from build123d import *

# Parameters (mm, degrees)
F0_R     = 2.5
F1_DEPTH = 15
F0_R_2   = 5
F0_R_3   = 3.5
F2_DEPTH = 2.5
F3_DEPTH = 9.5
F4_R     = 0.5
F5_R     = 0.5


with BuildPart() as f1:
    # F0 (on Front) → F1 (new body)
    with BuildSketch(Plane.XZ):
        Circle(F0_R)
    extrude(amount=F1_DEPTH)

    # F0 (on Front) → F2 (join)
    with BuildSketch(Plane.XZ):
        Circle(F0_R_2)
        Circle(F0_R_3, mode=Mode.SUBTRACT)
        Circle(F0_R_3)
        Circle(F0_R, mode=Mode.SUBTRACT)
        Circle(F0_R)
    extrude(amount=-F2_DEPTH)

    # F0 (on Front) → F3 (join)
    with BuildSketch(Plane.XZ):
        Circle(F0_R_3)
        Circle(F0_R, mode=Mode.SUBTRACT)
        Circle(F0_R)
    extrude(amount=-F3_DEPTH)

    # F4
    f4_edges = [f1.edges().sort_by_distance(p)[0] for p in [
        (-3.5, 9.5, 0),
    ]]
    fillet(f4_edges, radius=F4_R)

    # F5
    f5_edges = [f1.edges().sort_by_distance(p)[0] for p in [
        (-2.5, -15, 0),
    ]]
    fillet(f5_edges, radius=F5_R)


solid = f1.part
Check sheet for the modelled part. Datum: model origin and axes. Units: mm. A direction names the side the tool comes from. Coordinates: 2 decimals unless noted, no trailing zeros. Loops run counter-clockwise (first coordinate to the right, second up) from the corner with the lowest first, then second, coordinate; pieces in that order, holes last. Notation, with made-up numbers: (66, 30.25) -> (112, 30.25) arc R21 ccw to (112, 42.25) -> close; hole circle Ø6 at (-27, -1). An arc over 180 degrees is marked (long way). Answer in a Markdown table with one row per item.
1. Sectioned sample at A-A, the plane z = 0. Record the boundary of the cut face in (x, y).
Check values:
| item | result |
|---|---|
| outline | (-5, 0) -> (-2.5, 0) -> (-2.5, -14.5) arc R0.5 ccw to (-2, -15) -> (2, -15) arc R0.5 ccw to (2.5, -14.5) -> (2.5, 0) -> (5, 0) -> (5, 2.5) -> (3.5, 2.5) -> (3.5, 9) arc R0.5 ccw to (3, 9.5) -> (-3, 9.5) arc R0.5 ccw to (-3.5, 9) -> (-3.5, 2.5) -> (-5, 2.5) -> close |
2. Sectioned sample at B-B, the plane x = 0. Record the boundary of the cut face in (y, z).
Check values:
| item | result |
|---|---|
| outline | (-15, -2) arc R0.5 ccw to (-14.5, -2.5) -> (0, -2.5) -> (0, -5) -> (2.5, -5) -> (2.5, -3.5) -> (9, -3.5) arc R0.5 ccw to (9.5, -3) -> (9.5, 3) arc R0.5 ccw to (9, 3.5) -> (2.5, 3.5) -> (2.5, 5) -> (0, 5) -> (0, 2.5) -> (-14.5, 2.5) arc R0.5 ccw to (-15, 2) -> close |
3. Go/stop test with flat-tipped pins: pin 1 (1 mm diameter, centred on y = -4.5, z = 2, fed in from +X); pin 2 (2 mm diameter, centred on y = -10, z = -4, fed in from +X); pin 3 (1.5 mm diameter, centred on x = 3.5, z = 1.5, fed in from -Y). Record where each tip stops, or that it passes through.
Check values:
| item | result |
|---|---|
| pin 1 | stops at x = 2 |
| pin 2 | passes through |
| pin 3 | stops at y = 0 |
4. Material ranges on line 1 along Y through (x, z) = (0.25, -4.5); line 2 along Z through (x, y) = (-4, 2); line 3 along X through (y, z) = (-10, 1.5), recorded low to high. Write a range as [from, to].
Check values:
| item | result |
|---|---|
| line 1 | y = [0, 2.5] |
| line 2 | z = [-3, 3] |
| line 3 | x = [-2, 2] |
5. Access from +Z, -Z, +X, -X, +Y, -Y to the whole of each face (thin tool, end or side, straight path). Record for faces 1 (the face through (2.2, 2.5, -3.3)), 2 (the face through (2, 0, -2)), 3 (the face through (0, -15, 0)).
Check values:
| item | result |
|---|---|
| face 1 | +Y |
| face 2 | -Y |
| face 3 | +Z, -Z, +X, -X, -Y |
6. Sectioned sample at C-C, the plane y = 1.5. Record the boundary of the cut face in (x, z), then the cut area to 3 significant figures.
Check values:
| item | result |
|---|---|
| outline | circle Ø10 at (0, 0) |
| area | 78.5 mm2 |
7. Sectioned sample at D-D, the plane y = -3.5. Record the boundary of the cut face in (x, z).
Check values:
| item | result |
|---|---|
| outline | circle Ø5 at (0, 0) |
